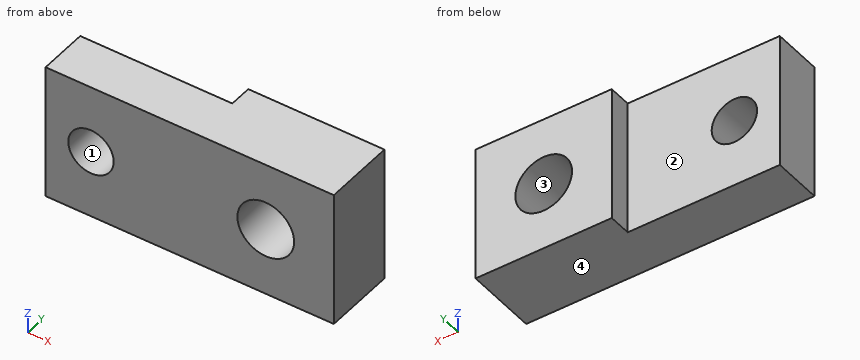
```python
from build123d import *

# Parameters (mm, degrees)
SKETCH1_W             = 12.7
SKETCH1_H             = 6
BOSS_EXTRUDE1_DEPTH   = 1.5875
M3X0_5_TAPPED_HOLE1_D = 2.5
SKETCH4_W             = 6.7
SKETCH4_H             = 1
CUT_EXTRUDE1_DEPTH    = 9.879338728
SKETCH5_R             = 1
CUT_EXTRUDE2_DEPTH    = 8.352083038


with BuildPart() as part:
    # Sketch1 → Boss-Extrude1 (new, symmetric)
    with BuildSketch(Plane(origin=(0, 0, 0), x_dir=(1, 0, 0), z_dir=(0, 1, 0))):
        Rectangle(SKETCH1_W, SKETCH1_H)
    extrude(amount=BOSS_EXTRUDE1_DEPTH, both=True)

    # M3x0.5 Tapped Hole1 (through all)
    with Locations(Plane(origin=(0, 1.5875, 0), x_dir=(1, 0, 0), z_dir=(0, 1, 0))):
        with Locations((3.35, 0)):
            Hole(M3X0_5_TAPPED_HOLE1_D / 2)

    # Sketch4 → Cut-Extrude1 (cut, through all)
    with BuildSketch(Plane.XY.offset(3)):
        with Locations((-3, 1.0875)):
            Rectangle(SKETCH4_W, SKETCH4_H)
    extrude(amount=-CUT_EXTRUDE1_DEPTH, mode=Mode.SUBTRACT)

    # Sketch5 → Cut-Extrude2 (cut, through all)
    with BuildSketch(Plane(origin=(0, 0.5875, 0), x_dir=(1, 0, 0), z_dir=(0, 1, 0))):
        with Locations(Location((-4.35, 0, 0), (0, 0, 270))):
            Circle(SKETCH5_R)
    extrude(amount=-CUT_EXTRUDE2_DEPTH, mode=Mode.SUBTRACT)


solid = part.part
```
Read the model definition and answer for the solid it produces. Units are mm, in the model's axes. Face numbers are marked on the shaded views. Give positions to 0.01 mm unless a question says otherwise; leave off trailing zeros. Write each loop counter-clockwise with the first axis right and the second up, starting at its lowest first coordinate (ties: lowest second). Pieces come first, ordered by that corner, then holes. Notation, with made-up numbers: (47, 36.25) -> (53, 36.25) arc R32 ccw to (53, 65.25) -> close; hole circle Ø11 at (69, -9.75). An arc over 180 degrees is marked (long way). Answer in a Markdown table with one row per item.
1) Section C-C on z = 0 is taken. Give the vertices of the cut face in (x, y), plus the area to 3 significant figures.
Results list:
| item | result |
|---|---|
| outline | (-6.35, -1.59) -> (-5.35, -1.59) -> (-5.35, 0.59) -> (-6.35, 0.59) -> close; (-3.35, -1.59) -> (2.1, -1.59) -> (2.1, 1.59) -> (0.35, 1.59) -> (0.35, 0.59) -> (-3.35, 0.59) -> close; (4.6, -1.59) -> (6.35, -1.59) -> (6.35, 1.59) -> (4.6, 1.59) -> close |
| area | 21.3 mm^2 |
2) Straight lines are drawn through the part: line 1 (Z direction, x = 3.35, y = 0.65); line 2 (X direction, y = 1.4, z = 0.4); line 3 (Y direction, x = 0.25, z = 2.3). For each, find the intervals that lie inside material, in ascending order. Write a range as [from, to].
Results list:
| item | result |
|---|---|
| line 1 | [-3, -1.25], [1.25, 3] |
| line 2 | [0.35, 2.17], [4.53, 6.35] |
| line 3 | [-1.59, 0.59] |
3) Section D-D on y = -0.25 is taken. Give the vertices of the cut face in (x, z).
Results list:
| item | result |
|---|---|
| outline | (-6.35, -3) -> (6.35, -3) -> (6.35, 3) -> (-6.35, 3) -> close; hole circle Ø2 at (-4.35, 0); hole circle Ø2.5 at (3.35, 0) |
4) Determine the mould class of the marked faces 1, 2, 3 and 4 for opening direction Z: released by +Z, released by -Z, zero draft, split by the parting line, or undercut.
Results list:
| item | result |
|---|---|
| face 1 | undercut |
| face 2 | zero draft |
| face 3 | undercut |
| face 4 | released by -Z |
5) Section B-B on y = 1.05 is taken. Give the vertices of the cut face in (x, z).
Results list:
| item | result |
|---|---|
| outline | (0.35, -3) -> (6.35, -3) -> (6.35, 3) -> (0.35, 3) -> close; hole circle Ø2.5 at (3.35, 0) |
6) Section A-A on x = -4.35 is taken. Give the vertices of the cut face in (y, z).
Results list:
| item | result |
|---|---|
| outline | (-1.59, -3) -> (0.59, -3) -> (0.59, -1) -> (-1.59, -1) -> close; (-1.59, 1) -> (0.59, 1) -> (0.59, 3) -> (-1.59, 3) -> close |
